Check sheet for the modelled part. Datum: model origin and axes. Units: mm. A direction names the side the tool comes from. Coordinates: 2 decimals unless noted, no trailing zeros. Loops run counter-clockwise (first coordinate to the right, second up) from the corner with the lowest first, then second, coordinate; pieces in that order, holes last.
```python
from build123d import *

# Parameters (mm, degrees)
Y_KSEKLIK_EKSTR_ZYON1_DEPTH = 2
IZIM2_W                     = 10
IZIM2_H                     = 2
Y_KSEKLIK_EKSTR_ZYON2_DEPTH = 10
IZIM3_R                     = 1.1
KES_EKSTR_ZYON1_DEPTH       = 30
IZIM4_W                     = 8
IZIM4_H                     = 3.5
KES_EKSTR_ZYON2_DEPTH       = 30
IZIM5_W                     = 5.5
IZIM5_H                     = 5.5
KES_EKSTR_ZYON3_DEPTH       = 1.2


with BuildPart() as part:
    # Çizim1 → Yükseklik-Ekstrüzyon1 (new body)
    with BuildSketch(Plane(origin=(0, 0, 0), x_dir=(1, 0, 0), z_dir=(0, 1, 0))):
        with BuildLine():
            Line((-12.738372093, 8.61627907), (22.261627907, 8.61627907))
            ThreePointArc((22.261627907, 8.61627907), (23.675841469, 8.030492632), (24.261627907, 6.61627907))
            Line((24.261627907, 6.61627907), (24.261627907, -13.38372093))
            ThreePointArc((24.261627907, -13.38372093), (23.675841469, -14.797934493), (22.261627907, -15.38372093))
            Line((22.261627907, -15.38372093), (-12.738372093, -15.38372093))
            ThreePointArc((-12.738372093, -15.38372093), (-14.152585655, -14.797934493), (-14.738372093, -13.38372093))
            Line((-14.738372093, -13.38372093), (-14.738372093, 6.61627907))
            ThreePointArc((-14.738372093, 6.61627907), (-14.152585655, 8.030492632), (-12.738372093, 8.61627907))
        make_face()
    extrude(amount=Y_KSEKLIK_EKSTR_ZYON1_DEPTH)

    # Çizim2 → Yükseklik-Ekstrüzyon2 (add)
    with BuildSketch(Plane(origin=(0, 2, 0), x_dir=(1, 0, 0), z_dir=(0, 1, 0))):
        with Locations((4.761627907, -12.28372093)):
            Rectangle(IZIM2_W, IZIM2_H)
        with Locations((4.761627907, 5.51627907)):
            Rectangle(IZIM2_W, IZIM2_H)
    extrude(amount=Y_KSEKLIK_EKSTR_ZYON2_DEPTH)

    # Çizim3 → Kes-Ekstrüzyon1 (cut)
    with BuildSketch(Plane.XY.offset(13.28372093)):
        with Locations((4.761627907, 7)):
            Circle(IZIM3_R)
    extrude(amount=-KES_EKSTR_ZYON1_DEPTH, mode=Mode.SUBTRACT)

    # Çizim4 → Kes-Ekstrüzyon2 (cut)
    with BuildSketch(Plane(origin=(0, 2, 0), x_dir=(1, 0, 0), z_dir=(0, 1, 0))):
        with Locations((-5.738372093, -3.38372093)):
            Rectangle(IZIM4_W, IZIM4_H)
    extrude(amount=-KES_EKSTR_ZYON2_DEPTH, mode=Mode.SUBTRACT)

    # Çizim5 → Kes-Ekstrüzyon3 (cut)
    with BuildSketch(Plane(origin=(0, 2, 0), x_dir=(1, 0, 0), z_dir=(0, 1, 0))):
        with Locations((15.511627907, -3.38372093)):
            Rectangle(IZIM5_W, IZIM5_H)
    extrude(amount=-KES_EKSTR_ZYON3_DEPTH, mode=Mode.SUBTRACT)


solid = part.part
```
1) Scan lines: line 1 (Z direction, x = 8, y = 7.75); line 2 (Y direction, x = -2, z = 11.25); line 3 (Y direction, x = 14.5, z = 4.75). Record each from-to range of solid material in increasing order.
Answer sheet:
line 1: z = -6.52 to -4.52, 11.28 to 13.28
line 2: y = 0 to 2
line 3: y = 0 to 0.8
2) Mould release check, pull along X, two halves, no side actions. Record for faces 1 (the flat face through (9.762, 7, -6)), 2 (the flat face through (5, 12, 12)), 3 (the flat face through (-0.238, 7, 12)), 4 (the flat face through (-9.738, 1, 3)): +X half, -X half, draft (parallel to the pull), parting line (faces both ways), or undercut.
Answer sheet:
face 1: +X half
face 2: draft
face 3: -X half
face 4: undercut
3) Section check C-C on y = 3. Enter the section's corners in (x, z), plus the area to 3 significant figures.
Answer sheet:
outline: (-0.24, -6.52) - (9.76, -6.52) - (9.76, -4.52) - (-0.24, -4.52) - close; (-0.24, 11.28) - (9.76, 11.28) - (9.76, 13.28) - (-0.24, 13.28) - close
area: 40.0 mm2
4) Section check A-A on y = 7. Enter the section's corners in (x, z), plus the area to 3 significant figures.
Answer sheet:
outline: (-0.24, -6.52) - (3.66, -6.52) - (3.66, -4.52) - (-0.24, -4.52) - close; (-0.24, 11.28) - (3.66, 11.28) - (3.66, 13.28) - (-0.24, 13.28) - close; (5.86, -6.52) - (9.76, -6.52) - (9.76, -4.52) - (5.86, -4.52) - close; (5.86, 11.28) - (9.76, 11.28) - (9.76, 13.28) - (5.86, 13.28) - close
area: 31.2 mm2
5) Set-up check for faces 5 (the flat face through (-1.738, 1, 3)), 6 (the flat face through (4, 6, 11.284)), 7 (the flat face through (5, 1, -8.616)), 8 (the flat face through (18.262, 1, 3)), 9 (the flat face through (4, 6, 13.284)): record each of +Z, -Z, +X, -X, +Y, -Y from which the full face is reachable in a straight line by a thin tool's end or side.
Answer sheet:
face 5: +Y, -Y
face 6: +X, -X, +Y
face 7: -Z, +X, -X, +Y, -Y
face 8: +Y
face 9: +Z, +X, -X, +Y
6) Depth check by flat-ended pin: pin 1 (3 mm diameter, centred on x = 19.5, z = 1.5, fed in from +Y); pin 2 (5 mm diameter, centred on y = 8, z = -4, fed in from +X); pin 3 (3 mm diameter, centred on x = 11, z = -5.5, fed in from +Y); pin 4 (3.5 mm diameter, centred on x = 4.76, y = 7, fed in from +Z). Enter the tip coordinate at first touch or a pass-through.
Answer sheet:
pin 1: stops at y = 2
pin 2: stops at x = 9.76
pin 3: stops at y = 12
pin 4: stops at z = 13.28
7) Section check D-D on z = 12.75. Enter the section's corners in (x, y).
Answer sheet:
outline: (-14.74, 0) - (24.26, 0) - (24.26, 2) - (9.76, 2) - (9.76, 12) - (-0.24, 12) - (-0.24, 2) - (-14.74, 2) - close; hole circle Ø2.2 at (4.76, 7)
8) Section check B-B on x = -3. Enter the section's corners in (y, z).
Answer sheet:
outline: (0, -8.62) - (2, -8.62) - (2, 1.63) - (0, 1.63) - close; (0, 5.13) - (2, 5.13) - (2, 15.38) - (0, 15.38) - close
